Could you check a few things on this model? Use its own coordinates, in mm. Give positions to 0.01 mm unless a question says otherwise; leave off trailing zeros. Answer in a Markdown table with one row per item.
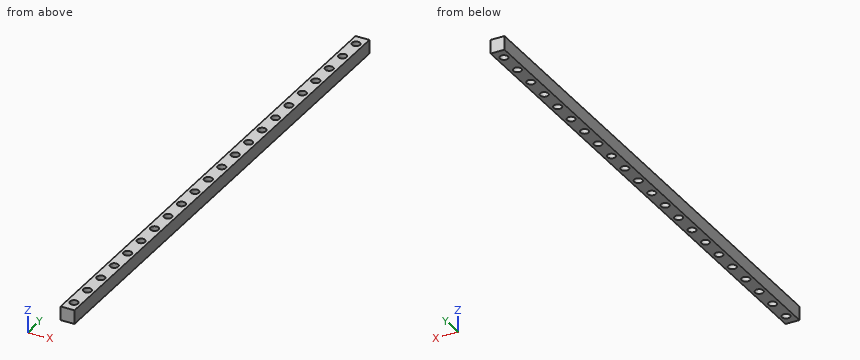
from build123d import *

# Parameters (mm, degrees)
SKETCH_W            = 6
SKETCH_H            = 6
PAD_DEPTH           = 230
SKETCH001_R         = 1.75
POCKET_DEPTH        = 6.001
LINEARPATTERN_COUNT = 22
LINEARPATTERN_PITCH = 10.47619


with BuildPart() as part:
    # Sketch → Pad (new body)
    with BuildSketch(Plane.XZ):
        Rectangle(SKETCH_W, SKETCH_H)
    extrude(amount=PAD_DEPTH)

    # Sketch001 → Pocket (cut, through all)
    with BuildSketch(Plane(origin=(0, 0, 3), x_dir=(-1, 0, 0), z_dir=(0, 0, 1))):
        with Locations((0, 5)):
            Circle(SKETCH001_R)
    pocket = extrude(amount=-POCKET_DEPTH, mode=Mode.SUBTRACT)

    # LinearPattern: Pocket ×22
    with Locations(*[(0, -i * LINEARPATTERN_PITCH, 0) for i in range(1, LINEARPATTERN_COUNT)]):
        add(pocket, mode=Mode.SUBTRACT)


solid = part.part
1) Imagine slicing it at A-A (x = 0). State how many separate pieces and enclosed holes the cut face has, then the cut area to 3 significant figures.
Check values:
| item | result |
|---|---|
| separate pieces | 23 |
| enclosed holes | 0 |
| area | 918 mm2 |
2) If I drill on line 1 (X direction, y = -141, z = 2); line 2 (X direction, y = -111, z = -1.85), over which ranges is the centre line in solid material (lowest first)?
Check values:
| item | result |
|---|---|
| line 1 | x = -3 to -1.74, 1.74 to 3 |
| line 2 | x = -3 to -1.24, 1.24 to 3 |
3) Will this pin go through, and if not, where does the flat tip stop? P1, Ø3, axis at x = 0, y = -120.24, coming from the +Z side.
Check values:
| item | result |
|---|---|
| P1 | passes through |
